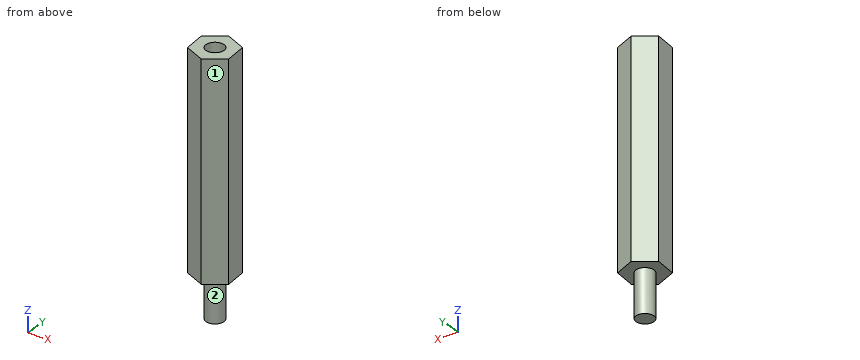
from build123d import *

# Parameters (mm, degrees)
BOSS_EXTRUDE1_DEPTH = 29.9466
SKETCH2_R           = 1.27
CUT_EXTRUDE1_DEPTH  = 24.8666
SKETCH3_R           = 1.27
BOSS_EXTRUDE2_DEPTH = 6.096


with BuildPart() as part:
    # Sketch1 → Boss-Extrude1 (new body)
    with BuildSketch(Plane.XY):
        Polygon((-2.597606711, -1.863500467), (0.315035389, -3.181343634), (2.912642099, -1.317843167), (2.597606711, 1.863500467), (-0.315035389, 3.181343634), (-2.912642099, 1.317843167), align=None)
    extrude(amount=BOSS_EXTRUDE1_DEPTH)

    # Sketch2 → Cut-Extrude1 (cut)
    with BuildSketch(Plane.XY.offset(29.9466)):
        Circle(SKETCH2_R)
    extrude(amount=-CUT_EXTRUDE1_DEPTH, mode=Mode.SUBTRACT)

    # Sketch3 → Boss-Extrude2 (add)
    with BuildSketch(Plane(origin=(0, 0, 0), x_dir=(-1, 0, 0), z_dir=(0, 0, -1))):
        with Locations(Location((0, 0, 0), (0, 0, 180))):
            Circle(SKETCH3_R)
    extrude(amount=BOSS_EXTRUDE2_DEPTH)


solid = part.part
Verification items for the finished model (mm, model axes). Face numbers are marked on the shaded views. A direction names the side the tool comes from. Coordinates: 2 decimals unless noted, no trailing zeros. Order: outer loops, then holes, each group sorted by start corner. A loop starts at its lowest first (then second) coordinate and runs counter-clockwise, first axis right, second up. Notation, with made-up numbers: (-26.5, 82.5) -> (1.5, 82.5) arc R26 cw to (1.5, 107.5) -> close; hole circle Ø10 at (2.5, 0). An arc over 180 degrees is marked (long way). Use CSV: the item, a comma, the result in double quotes. Start each with the question number.
Q1. Section check D-D, the plane x = 1.75. Record the cut outline in (y, z).
Q2. Section check B-B, the plane x = -0.7. Record the cut outline in (y, z), and give its area (3 significant figures).
Q3. Thickness scan on line 1 along Z through (x, y) = (-0.65, 0.5); line 2 along X through (y, z) = (1, 25.5); line 3 along X through (y, z) = (-0.25, 27.5). Record the ranges inside material, lowest first.
Q4. Depth check by flat-ended pin: P1, Ø1, axis at x = -2, z = 24, coming from the -Y side; P2, Ø1, axis at x = 1.5, z = 10.5, coming from the -Y side; P3, Ø3, axis at y = -2, z = 0.5, coming from the -X side. Enter the tip coordinate at first touch or a pass-through.
Q5. Section check C-C, the plane y = 0. Record the cut outline in (x, z), and give its area (3 significant figures).
Q6. Section check A-A, the plane z = 22. Record the cut outline in (x, y), and give its area (3 significant figures).
Q7. Tool access check on the marked faces 1 and 2. Record the directions out of +Z, -Z, +X, -X, +Y, -Y that give a thin tool (end or side, any length) a straight path to the whole face; none if there is none.
Returned:
1,outline,"(-2.15, 0) -> (2.25, 0) -> (2.25, 29.95) -> (-2.15, 29.95) -> close"
2,outline,"(-2.72, 0) -> (-1.06, 0) -> (-1.06, -6.1) -> (1.06, -6.1) -> (1.06, 0) -> (2.91, 0) -> (2.91, 29.95) -> (1.06, 29.95) -> (1.06, 5.08) -> (-1.06, 5.08) -> (-1.06, 29.95) -> (-2.72, 29.95) -> close"
2,area,"129 mm^2"
3,line 1,"z = -6.1 to 5.08"
3,line 2,"x = -2.88 to -0.78, 0.78 to 2.68"
3,line 3,"x = -2.76 to -1.25, 1.25 to 2.81"
4,P1,"stops at y = -2.36"
4,P2,"stops at y = -2.69"
4,P3,"stops at x = -2.73"
5,outline,"(-2.78, 0) -> (-1.27, 0) -> (-1.27, -6.1) -> (1.27, -6.1) -> (1.27, 0) -> (2.78, 0) -> (2.78, 29.95) -> (1.27, 29.95) -> (1.27, 5.08) -> (-1.27, 5.08) -> (-1.27, 29.95) -> (-2.78, 29.95) -> close"
5,area,"119 mm^2"
6,outline,"(-2.91, 1.32) -> (-2.6, -1.86) -> (0.32, -3.18) -> (2.91, -1.32) -> (2.6, 1.86) -> (-0.32, 3.18) -> close; hole circle Ø2.54 at (0, 0)"
6,area,"21.5 mm^2"
7,face 1,"+Z, -Z, +X, -Y"
7,face 2,"-Z"
